Geometry check sheet. Reference: the model listing, model coordinates, mm. Face numbers are marked on the shaded views. A direction names the side the tool comes from. Coordinates: 2 decimals unless noted, no trailing zeros. Order: outer loops, then holes, each group sorted by start corner. A loop starts at its lowest first (then second) coordinate and runs counter-clockwise, first axis right, second up. Notation, with made-up numbers: M 63,-7.75 L 116,-7.75 A18 ccw 116,10.25 Z; hole C 10.25,-35 d6. An arc over 180 degrees is marked long. Use CSV: the item, a comma, the result in double quotes. Start each with the question number.
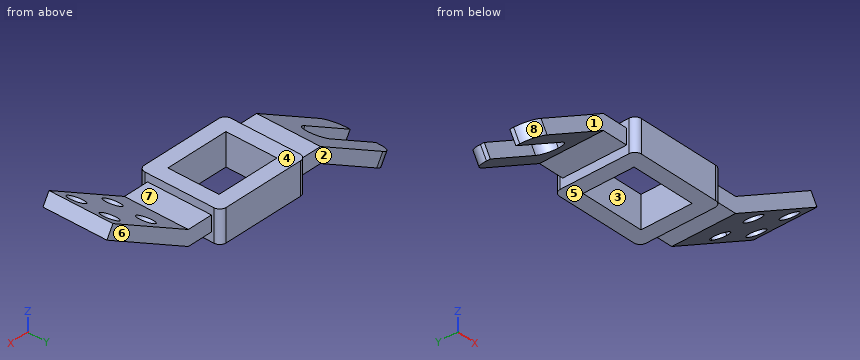
```python
from build123d import *

# Parameters (mm, degrees)
F0_W           = 74
F0_H           = 64
F0_W_2         = 50
F0_H_2         = 40
F1_DEPTH       = 25
F2_W           = 50
F2_H           = 12
F3_DEPTH       = 20
F5_DEPTH       = 25
F5_DEPTH_BACK  = 25
F7_DEPTH       = 25
F8_W           = 50
F8_H           = 12
F9_DEPTH       = 20
F10_W          = 20
F10_H          = 12
F11_DEPTH      = 25
F11_DEPTH_BACK = 25
F12_R          = 6.5
F13_DEPTH      = 25
F14_R          = 5
F15_R          = 12


with BuildPart() as f1:
    # F0 (on Top) → F1 (new body)
    with BuildSketch(Plane.XY):
        Rectangle(F0_W, F0_H)
        Rectangle(F0_W_2, F0_H_2, mode=Mode.SUBTRACT)
    extrude(amount=F1_DEPTH)

    # F2 (on face) → F3 (join)
    with BuildSketch(Plane(origin=(-37, 0, 0), x_dir=(0, -1, 0), z_dir=(-1, 0, 0))):
        with Locations((0, 13)):
            Rectangle(F2_W, F2_H)
    extrude(amount=F3_DEPTH)

    # F4 (on Front) → F5 (join, two sides)
    with BuildSketch(Plane.XZ) as f5_sk:
        Polygon((-115.8897274573, -27), (-57, 7), (-57, 19), (-121.08587988, -18), align=None)
    extrude(amount=F5_DEPTH)
    extrude(f5_sk.sketch, amount=-F5_DEPTH_BACK)

    # F6 (on face) → F7 (cut)
    with BuildSketch(Plane(origin=(-22.477241336, 0, 38.9317240079), x_dir=(0.8660254038, 0, 0.5), z_dir=(-0.5, 0, 0.8660254038))):
        with BuildLine():
            ThreePointArc((-68.8634480157, -10), (-61.7923802038, -7.0710678119), (-58.8634480157, 0))
            Line((-58.8634480157, 0), (-78.8634480157, 0))
            ThreePointArc((-78.8634480157, 0), (-75.9345158276, -7.0710678119), (-68.8634480157, -10))
        make_face()
        with BuildLine():
            Line((-78.8634480157, 0), (-58.8634480157, 0))
            ThreePointArc((-58.8634480157, 0), (-61.7923802038, 7.0710678119), (-68.8634480157, 10))
            ThreePointArc((-68.8634480157, 10), (-75.9345158276, 7.0710678119), (-78.8634480157, 0))
        make_face()
        with BuildLine():
            ThreePointArc((-68.8634480157, -10), (-75.9345158276, -7.0710678119), (-78.8634480157, 0))
            Line((-78.8634480157, 0), (-113.8634480157, 0))
            Line((-113.8634480157, 0), (-113.8634480157, -10))
            Line((-113.8634480157, -10), (-68.8634480157, -10))
        make_face()
        with BuildLine():
            Line((-113.8634480157, 0), (-78.8634480157, 0))
            ThreePointArc((-78.8634480157, 0), (-75.9345158276, 7.0710678119), (-68.8634480157, 10))
            Line((-68.8634480157, 10), (-113.8634480157, 10))
            Line((-113.8634480157, 10), (-113.8634480157, 0))
        make_face()
    extrude(amount=-F7_DEPTH, mode=Mode.SUBTRACT)

    # F8 (on face) → F9 (join)
    with BuildSketch(Plane.YZ.offset(37)):
        with Locations((0, 13)):
            Rectangle(F8_W, F8_H)
    extrude(amount=F9_DEPTH)

    # F10 (on Front) → F11 (join, two sides)
    with BuildSketch(Plane.XZ) as f11_sk:
        with Locations((47, 13)):
            Rectangle(F10_W, F10_H)
        Polygon((121.9519052838, 56.5), (57, 19), (57, 7), (127.1480577065, 47.5), align=None)
    extrude(amount=F11_DEPTH)
    extrude(f11_sk.sketch, amount=-F11_DEPTH_BACK)

    # F12 (on face) → F13 (cut)
    with BuildSketch(Plane(origin=(6.022758664, 0, -10.4317240079), x_dir=(0.8660254038, 0, 0.5), z_dir=(-0.5, 0, 0.8660254038))):
        with BuildLine():
            ThreePointArc((92.3634480157, 13), (90.4596420934, 17.5961940777), (85.8634480157, 19.5))
            ThreePointArc((85.8634480157, 19.5), (81.267253938, 8.4038059223), (92.3634480157, 13))
        make_face()
        with Locations((121.8634480157, 13)):
            Circle(F12_R)
        with Locations((121.8634480157, -13)):
            Circle(F12_R)
        with Locations((85.8634480157, -13)):
            Circle(F12_R)
    extrude(amount=-F13_DEPTH, mode=Mode.SUBTRACT)

    # F14
    f14_edges = [f1.edges().sort_by_distance(p)[0] for p in [
        (-37, 32, 12.5),
        (37, 32, 12.5),
        (-37, -32, 12.5),
        (37, -32, 12.5),
    ]]
    fillet(f14_edges, radius=F14_R)

    # F15
    f15_edges = [f1.edges().sort_by_distance(p)[0] for p in [
        (-118.487804, 25, -22.5),
        (-118.487804, -25, -22.5),
    ]]
    fillet(f15_edges, radius=F15_R)


solid = f1.part
```
1) Draft check along X on the marked faces 6, 7 and 8. Enter one of: +X half, -X half, draft (parallel to the pull), parting line (faces both ways), or undercut.
2) Gauge pin test, flat ends, axial feed: P1, Ø7.5, axis at y = 11, z = 12, coming from the -X side; P2, Ø6, axis at x = -57.5, z = 17, coming from the -Y side; P3, Ø22, axis at x = 50.5, y = 7, coming from the +Z side. Record the tip position at first contact, or that the pin passes through.
3) Section check B-B on y = 4. Record the boundary of the cut face in (x, z).
4) Section check A-A on x = 6. Record the boundary of the cut face in (y, z), then the cut area to 3 significant figures.
5) Section check D-D on y = 22.5. Record the boundary of the cut face in (x, z), then the cut area to 3 significant figures.
6) Section check C-C on x = -89. Record the boundary of the cut face in (y, z), then the cut area to 3 significant figures.
7) Set-up check for the marked faces 1, 2, 3, 4 and 5: record each of +Z, -Z, +X, -X, +Y, -Y from which the full face is reachable in a straight line by a thin tool's end or side.
8) Material ranges on line 1 along X through (y, z) = (-9.5, 20); line 2 along Y through (x, z) = (-9.5, 22); line 3 along Y through (x, z) = (-88.5, -2), recorded low to high.
Results are:
1,face 6,"draft"
1,face 7,"undercut"
1,face 8,"-X half"
2,P1,"stops at x = -75.62"
2,P2,"stops at y = -25"
2,P3,"stops at z = 21.6"
3,outline,"M -74.18,9.08 L -68.98,0.08 L -57,7 L -37,7 L -37,0 L -25,0 L -25,25 L -37,25 L -37,19 L -57,19 Z; M 25,0 L 37,0 L 37,7 L 57,7 L 127.15,47.5 L 121.95,56.5 L 57,19 L 37,19 L 37,25 L 25,25 Z"
4,outline,"M -32,0 L -20,0 L -20,25 L -32,25 Z; M 20,0 L 32,0 L 32,25 L 20,25 Z"
4,area,"600 mm²"
5,outline,"M -117.04,-15.67 L -111.85,-24.67 L -57,7 L -37,7 L -37,0 L 37,0 L 37,7 L 57,7 L 127.15,47.5 L 121.95,56.5 L 57,19 L 37,19 L 37,25 L -37,25 L -37,19 L -57,19 Z"
5,area,"3,830 mm²"
6,outline,"M -25,-11.48 L -10,-11.48 L -10,0.52 L -25,0.52 Z; M 10,-11.48 L 25,-11.48 L 25,0.52 L 10,0.52 Z"
6,area,"360 mm²"
7,face 1,"+Z, -Z, -X, -Y"
7,face 2,"+Z, -Z, -X, +Y"
7,face 3,"+Z, -Z"
7,face 4,"+Z, -X, +Y, -Y"
7,face 5,"-Z, +X, +Y, -Y"
8,line 1,"x = -37 to -25, 25 to 37, 58.73 to 79.52"
8,line 2,"y = -32 to -20, 20 to 32"
8,line 3,"y = -25 to -10, 10 to 25"
